Build history of the part. All positions in model axes, mm. Round coordinates to 2 decimals unless told otherwise and drop trailing zeros. Loops run counter-clockwise (first coordinate to the right, second up) from the corner with the lowest first, then second, coordinate; pieces in that order, holes last. Notation, with made-up numbers: (-29.75, -25) - (10.25, -25) arc R20 ccw to (10.25, -20) - close; hole circle Ø11 at (-1, 30.5). An arc over 180 degrees is marked (long way). One line per question, with ' | ' between items. Start each with the question number.
from build123d import *

# Parameters (mm, degrees)
SKETCH006_R     = 43
SKETCH006_R_2   = 1.5
SKETCH006_R_3   = 4
PAD_DEPTH       = 4
CHAMFER001_SIZE = 1.9


with BuildPart() as part:
    # Sketch006 → Pad (new body)
    with BuildSketch(Plane.XY.offset(22)):
        Circle(SKETCH006_R)
        with Locations((0, 36)):
            Circle(SKETCH006_R_2, mode=Mode.SUBTRACT)
        with Locations((31.176915, -18)):
            Circle(SKETCH006_R_2, mode=Mode.SUBTRACT)
        with Locations((-31.176915, -18)):
            Circle(SKETCH006_R_2, mode=Mode.SUBTRACT)
        Circle(SKETCH006_R_3, mode=Mode.SUBTRACT)
    extrude(amount=PAD_DEPTH)

    # Chamfer001
    chamfer001_edges = [part.edges().sort_by_distance(p)[0] for p in [
        (-32.676915, -18, 22),
        (29.676915, -18, 22),
        (-1.5, 36, 22),
    ]]
    chamfer(chamfer001_edges, length=CHAMFER001_SIZE)


solid = part.part
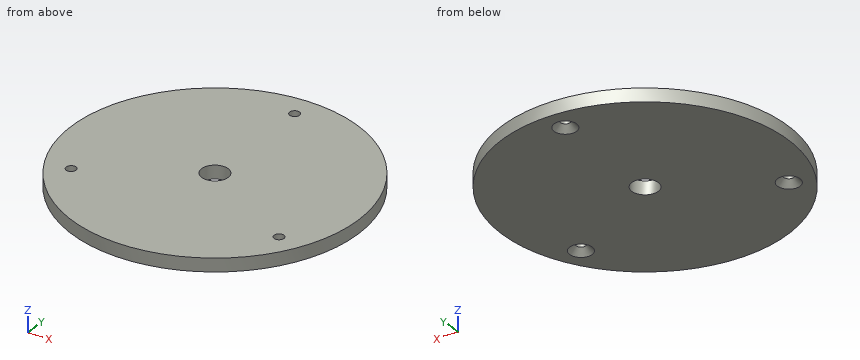
1) Saw through at C-C on z = 24.65. Write the cut outline in (x, y), and give its area (3 significant figures).
2) Wall check: line 1 (Y direction, x = -31.5, z = 25.85); line 2 (X direction, y = 36, z = 23.5); line 3 (Y direction, x = 24, z = 23.45). Give the ranges that are in metal, low to high. Write a range as [from, to].
3) Saw through at A-A on x = 0. Write the cut outline in (y, z).
4) Saw through at B-B on y = 0. Write the cut outline in (x, z).
5) Saw through at D-D on y = -18. Write the cut outline in (x, z).
6) Drop flat-ended pins along their axis: pin 1 (1.5 mm diameter, centred on x = -14, z = 24.5, fed in from -Y); pin 2 (1.5 mm diameter, centred on y = 19.5, z = 25.5, fed in from +X); pin 3 (1.5 mm diameter, centred on x = 9, z = 24, fed in from -Y). Give the stop position or say it passes through.
Answer key:
1) outline: circle Ø86 at (0, 0); hole circle Ø3 at (-31.18, -18); hole circle Ø8 at (0, 0); hole circle Ø3 at (0, 36); hole circle Ø3 at (31.18, -18) | area: 5,740 mm²
2) line 1: [-29.27, -19.46], [-16.54, 29.27] | line 2: [-23.52, -1.9], [1.9, 23.52] | line 3: [-35.68, 35.68]
3) outline: (-43, 22) - (-4, 22) - (-4, 26) - (-43, 26) - close; (4, 22) - (32.6, 22) - (34.5, 23.9) - (34.5, 26) - (4, 26) - close; (37.5, 23.9) - (39.4, 22) - (43, 22) - (43, 26) - (37.5, 26) - close
4) outline: (-43, 22) - (-4, 22) - (-4, 26) - (-43, 26) - close; (4, 22) - (43, 22) - (43, 26) - (4, 26) - close
5) outline: (-39.05, 22) - (-34.58, 22) - (-32.68, 23.9) - (-32.68, 26) - (-39.05, 26) - close; (-29.68, 23.9) - (-27.78, 22) - (27.78, 22) - (29.68, 23.9) - (29.68, 26) - (-29.68, 26) - close; (32.68, 23.9) - (34.58, 22) - (39.05, 22) - (39.05, 26) - (32.68, 26) - close
6) pin 1: y = -40.91 | pin 2: x = 38.7 | pin 3: y = -42.2
